Read the model definition and answer for the solid it produces. Units are mm, in the model's axes. A direction names the side the tool comes from. Give positions to 0.01 mm unless a question says otherwise; leave off trailing zeros. Order: outer loops, then holes, each group sorted by start corner. A loop starts at its lowest first (then second) coordinate and runs counter-clockwise, first axis right, second up. Notation, with made-up numbers: M 87,-18.75 L 109,-18.75 A20 ccw 109,-8.75 Z; hole C -32,37 d1. An arc over 180 degrees is marked long. One line per item, written item: value.
from build123d import *

# Parameters (mm, degrees)
SKETCH_1_W          = 20
SKETCH_1_H          = 20
SKETCH_1_W_2        = 16
SKETCH_1_H_2        = 16
EXTRUDE_1_DEPTH     = 400
SKETCH_9_R          = 1.5
CUT_EXTRUDE_6_DEPTH = 401.998753115
SKETCH_10_R         = 7.5
CUT_EXTRUDE_7_DEPTH = 401.998753115
SKETCH_11_R         = 1.5
CUT_EXTRUDE_8_DEPTH = 401.998753115


with BuildPart() as part:
    # 草图1 → 凸台-拉伸1 (new body)
    with BuildSketch(Plane.XY):
        with Locations((10, 10)):
            Rectangle(SKETCH_1_W, SKETCH_1_H)
        with Locations((10, 10)):
            Rectangle(SKETCH_1_W_2, SKETCH_1_H_2, mode=Mode.SUBTRACT)
    extrude(amount=EXTRUDE_1_DEPTH)

    # 草图9 → 切除-拉伸6 (cut, through all)
    with BuildSketch(Plane(origin=(0, 20, 0), x_dir=(1, 0, 0), z_dir=(0, 1, 0))):
        with Locations(Location((10, -390, 0), (0, 0, 270))):
            Circle(SKETCH_9_R)
        with Locations(Location((10, -380, 0), (0, 0, 270))):
            Circle(SKETCH_9_R)
        with Locations(Location((10, -370, 0), (0, 0, 270))):
            Circle(SKETCH_9_R)
        with Locations(Location((10, -360, 0), (0, 0, 270))):
            Circle(SKETCH_9_R)
        with Locations(Location((10, -350, 0), (0, 0, 270))):
            Circle(SKETCH_9_R)
        with Locations(Location((10, -340, 0), (0, 0, 270))):
            Circle(SKETCH_9_R)
        with Locations(Location((10, -330, 0), (0, 0, 270))):
            Circle(SKETCH_9_R)
        with Locations(Location((10, -320, 0), (0, 0, 270))):
            Circle(SKETCH_9_R)
        with Locations(Location((10, -310, 0), (0, 0, 270))):
            Circle(SKETCH_9_R)
        with Locations(Location((10, -300, 0), (0, 0, 270))):
            Circle(SKETCH_9_R)
        with Locations(Location((10, -290, 0), (0, 0, 270))):
            Circle(SKETCH_9_R)
        with Locations(Location((10, -280, 0), (0, 0, 270))):
            Circle(SKETCH_9_R)
        with Locations(Location((10, -270, 0), (0, 0, 270))):
            Circle(SKETCH_9_R)
        with Locations(Location((10, -260, 0), (0, 0, 270))):
            Circle(SKETCH_9_R)
        with Locations(Location((10, -250, 0), (0, 0, 270))):
            Circle(SKETCH_9_R)
        with Locations(Location((10, -240, 0), (0, 0, 270))):
            Circle(SKETCH_9_R)
        with Locations(Location((10, -230, 0), (0, 0, 270))):
            Circle(SKETCH_9_R)
        with Locations(Location((10, -220, 0), (0, 0, 270))):
            Circle(SKETCH_9_R)
        with Locations(Location((10, -210, 0), (0, 0, 270))):
            Circle(SKETCH_9_R)
        with Locations(Location((10, -200, 0), (0, 0, 270))):
            Circle(SKETCH_9_R)
        with Locations(Location((10, -190, 0), (0, 0, 270))):
            Circle(SKETCH_9_R)
        with Locations(Location((10, -180, 0), (0, 0, 270))):
            Circle(SKETCH_9_R)
        with Locations(Location((10, -170, 0), (0, 0, 270))):
            Circle(SKETCH_9_R)
        with Locations(Location((10, -160, 0), (0, 0, 270))):
            Circle(SKETCH_9_R)
        with Locations(Location((10, -150, 0), (0, 0, 270))):
            Circle(SKETCH_9_R)
        with Locations(Location((10, -140, 0), (0, 0, 270))):
            Circle(SKETCH_9_R)
        with Locations(Location((10, -130, 0), (0, 0, 270))):
            Circle(SKETCH_9_R)
        with Locations(Location((10, -120, 0), (0, 0, 270))):
            Circle(SKETCH_9_R)
        with Locations(Location((10, -110, 0), (0, 0, 270))):
            Circle(SKETCH_9_R)
        with Locations(Location((10, -100, 0), (0, 0, 270))):
            Circle(SKETCH_9_R)
        with Locations(Location((10, -90, 0), (0, 0, 270))):
            Circle(SKETCH_9_R)
        with Locations(Location((10, -80, 0), (0, 0, 270))):
            Circle(SKETCH_9_R)
        with Locations(Location((10, -70, 0), (0, 0, 270))):
            Circle(SKETCH_9_R)
        with Locations(Location((10, -60, 0), (0, 0, 270))):
            Circle(SKETCH_9_R)
        with Locations(Location((10, -50, 0), (0, 0, 270))):
            Circle(SKETCH_9_R)
        with Locations(Location((10, -40, 0), (0, 0, 270))):
            Circle(SKETCH_9_R)
        with Locations(Location((10, -30, 0), (0, 0, 270))):
            Circle(SKETCH_9_R)
        with Locations(Location((10, -20, 0), (0, 0, 270))):
            Circle(SKETCH_9_R)
        with Locations(Location((10, -10, 0), (0, 0, 270))):
            Circle(SKETCH_9_R)
    extrude(amount=-CUT_EXTRUDE_6_DEPTH, mode=Mode.SUBTRACT)

    # 草图10 → 切除-拉伸7 (cut, through all)
    with BuildSketch(Plane(origin=(20, 0, 0), x_dir=(0, 0, -1), z_dir=(1, 0, 0))):
        with Locations((-365, 10)):
            Circle(SKETCH_10_R)
        with Locations((-35, 10)):
            Circle(SKETCH_10_R)
    extrude(amount=-CUT_EXTRUDE_7_DEPTH, mode=Mode.SUBTRACT)

    # 草图11 → 切除-拉伸8 (cut, through all)
    with BuildSketch(Plane(origin=(20, 0, 0), x_dir=(0, 0, -1), z_dir=(1, 0, 0))):
        with Locations((-315, 14)):
            Circle(SKETCH_11_R)
        with Locations((-300, 14)):
            Circle(SKETCH_11_R)
        with Locations((-300, 4)):
            Circle(SKETCH_11_R)
        with Locations((-315, 4)):
            Circle(SKETCH_11_R)
        with Locations(Location((-85, 4, 0), (0, 0, 180))):
            Circle(SKETCH_11_R)
        with Locations(Location((-100, 4, 0), (0, 0, 180))):
            Circle(SKETCH_11_R)
        with Locations(Location((-100, 14, 0), (0, 0, 180))):
            Circle(SKETCH_11_R)
        with Locations(Location((-85, 14, 0), (0, 0, 180))):
            Circle(SKETCH_11_R)
    extrude(amount=-CUT_EXTRUDE_8_DEPTH, mode=Mode.SUBTRACT)


solid = part.part
1) Consider probe 1 along Y at (x, z) = (19.2, 100); probe 2 along X at (y, z) = (2.75, 377). Determine where each line is inside the solid, lowest interval first.
Reported:
probe 1: y = 0 to 2.5, 5.5 to 12.5, 15.5 to 20
probe 2: x = 0 to 2, 18 to 20
2) This flat-tipped pin is pushed along its axis until it touches: pin 1 Ø2.5 at (x, z) = (10, 360) entering from -Y. Where does it stop, or does it pass through?
Reported:
pin 1: passes through
3) Find section A-A, the plane z = 365. Write down the section's boundary in (x, y).
Reported:
outline: M 0,0 L 20,0 L 20,2.5 L 18,2.5 L 18,2 L 2,2 L 2,2.5 L 0,2.5 Z; M 0,17.5 L 2,17.5 L 2,18 L 18,18 L 18,17.5 L 20,17.5 L 20,20 L 0,20 Z
4) Which of the six approach directions +Z, -Z, +X, -X, +Y, -Y give full straight-line access (tool end or side, diameter ignored) to faces 5 (the face through (10, 2, 197)), 6 (the face through (1, 10, 400))?
Reported:
face 5: +Z, -Z
face 6: +Z, +X, -X, +Y, -Y
5) Determine the mould class of faces 1 (the face through (18, 10, 197)), 2 (the face through (10, 20, 197)), 3 (the face through (0, 10, 197)), 4 (the face through (2, 10, 197)) for opening direction X: +X half, -X half, draft (parallel to the pull), parting line (faces both ways), or undercut.
Reported:
face 1: undercut
face 2: draft
face 3: -X half
face 4: undercut
